Answer from the drawing. Dimensions are ordinates in mm from the lowest x, y and z of the part. A direction names the side the tool comes from. Coordinates: 2 decimals unless noted, no trailing zeros. Loops run counter-clockwise (first coordinate to the right, second up) from the corner with the lowest first, then second, coordinate; pieces in that order, holes last.
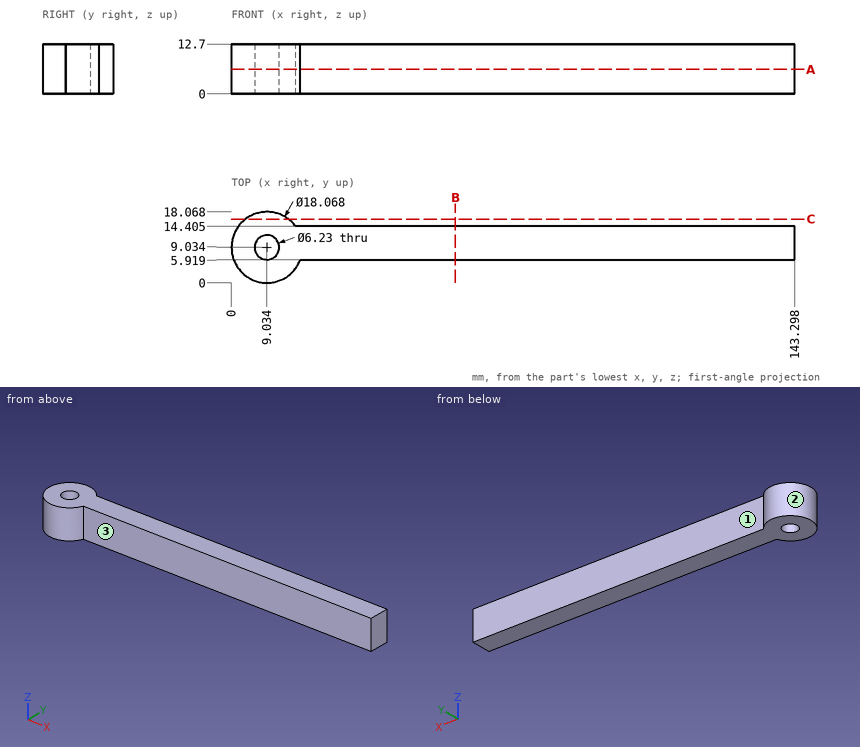
Item 1: Which of the six approach directions +Z, -Z, +X, -X, +Y, -Y give full straight-line access (tool end or side, diameter ignored) to the marked faces 1, 2 and 3?
Numbers:
face 1: +Z, -Z, +X, +Y
face 2: +Z, -Z
face 3: +Z, -Z, +X, -Y
Item 2: Given pin 1 (6.5 mm diameter, centred on x = 89.5, z = 6.5, fed in from +Y) (1 decimal); pin 2 (1 mm diameter, centred on y = 5, z = 8.5, fed in from +X); pin 3 (3 mm diameter, centred on x = 89.5, z = 6, fed in from -Y), each flat-ended and moving along its own axis, determine where each tip first touches the part or whether it passes through.
Numbers:
pin 1: stops at y = 14.4
pin 2: stops at x = 17.35
pin 3: stops at y = 5.92
Item 3: Find the intervals of material crossed by line 1 along X through (y, z) = (10, 3) (1 decimal); line 2 along Y through (x, z) = (136, 1) (1 decimal); line 3 along X through (y, z) = (6.5, 12) (1 decimal), in increasing order.
Numbers:
line 1: x = 0.1 to 6.1, 12 to 143.3
line 2: y = 5.9 to 14.4
line 3: x = 0.4 to 7.2, 10.8 to 143.3
Item 4: A cutting plane is placed at B-B on x = 57. Determine the outline of the cut face in (y, z) (1 decimal), then the cut area to 3 significant figures.
Numbers:
outline: (5.9, 0) - (14.4, 0) - (14.4, 12.7) - (5.9, 12.7) - close
area: 108 mm2
Item 5: A cutting plane is placed at A-A on z = 6.25. Determine the outline of the cut face in (x, y) (1 decimal), then the cut area to 3 significant figures.
Numbers:
outline: (16.3, 14.4) arc R9 ccw (long way) to (17.5, 5.9) - (143.3, 5.9) - (143.3, 14.4) - close; hole circle Ø6.2 at (9, 9)
area: 1,290 mm2
Item 6: A cutting plane is placed at C-C on y = 16.25. Determine the outline of the cut face in (x, z), then the cut area to 3 significant figures.
Numbers:
outline: (3.6, 0) - (14.47, 0) - (14.47, 12.7) - (3.6, 12.7) - close
area: 138 mm2
